from build123d import *

# Parameters (mm, degrees)
SKETCH_1_W          = 15.4
SKETCH_1_H          = 22.4
EXTRUDE_2_DEPTH     = 3
EXTRUDE_3_DEPTH     = 10
EXTRUDE_3_2_DEPTH   = 10
EXTRUDE_4_DEPTH     = 15
SKETCH_3_R          = 1.6
CUT_EXTRUDE_2_DEPTH = 31.8
SKETCH_9_R          = 1.3
SKETCH_9_R_2        = 3
SKETCH_9_R_3        = 1.55
CUT_EXTRUDE_6_DEPTH = 16
SKETCH_10_R         = 2.9
CUT_EXTRUDE_7_DEPTH = 2


with BuildPart() as part:
    # Sketch 1 → Extrude 2 (new body)
    with BuildSketch(Plane(origin=(0, 0, 0), x_dir=(1, 0, 0), z_dir=(0, 1, 0))):
        Rectangle(SKETCH_1_W, SKETCH_1_H)
    extrude(amount=EXTRUDE_2_DEPTH)



with BuildPart() as body_2:
    # Sketch 1_4 → Extrude 3 (new body)
    with BuildSketch(Plane(origin=(0, 0, 0), x_dir=(1, 0, 0), z_dir=(0, 1, 0))):
        Polygon((7.7, -11.2), (7.7, -7.7), (0, -7.7), (-4.7, -7.7), (-7.7, -7.7), (-7.7, -11.2), align=None)
    extrude(amount=EXTRUDE_3_DEPTH)


with BuildPart() as body_3:
    # Sketch 1_4 → Extrude 3 2 (new body)
    with BuildSketch(Plane(origin=(0, 0, 0), x_dir=(1, 0, 0), z_dir=(0, 1, 0))):
        Polygon((-7.7, 7.7), (0, 7.7), (7.7, 7.7), (7.7, 11.2), (-7.7, 11.2), align=None)
    extrude(amount=EXTRUDE_3_2_DEPTH)


with BuildPart() as part_1:
    add(part.part)

    add(body_2.part)  # Extrude 4 merges body 2

    add(body_3.part)  # Extrude 4 merges body 3
    # Sketch 1_5 → Extrude 4 (add)
    with BuildSketch(Plane(origin=(0, 0, 0), x_dir=(1, 0, 0), z_dir=(0, 1, 0))):
        Polygon((-7.7, 0), (-7.7, 7.7), (-7.7, 11.2), (-13.2, 11.2), (-13.2, -11.2), (-7.7, -11.2), (-7.7, -7.7), align=None)
        Polygon((7.7, 11.2), (7.7, 7.7), (7.7, 0), (7.7, -7.7), (7.7, -11.2), (13.2, -11.2), (13.2, 11.2), align=None)
        Polygon((7.7, -11.2), (7.7, -7.7), (0, -7.7), (-4.7, -7.7), (-7.7, -7.7), (-7.7, -11.2), align=None)
        Polygon((-7.7, 7.7), (0, 7.7), (7.7, 7.7), (7.7, 11.2), (-7.7, 11.2), align=None)
    extrude(amount=EXTRUDE_4_DEPTH)

    # Sketch 3 → Cut-Extrude 2 (cut, through all)
    with BuildSketch(Plane(origin=(0, 0, -19.6), x_dir=(-1, 0, 0), z_dir=(0, 0, -1))):
        with Locations((0, 3)):
            Circle(SKETCH_3_R)
        with Locations((-10, 3)):
            Circle(SKETCH_3_R)
        with Locations((10, 3)):
            Circle(SKETCH_3_R)
    extrude(amount=-CUT_EXTRUDE_2_DEPTH, mode=Mode.SUBTRACT)

    # Sketch 9 → Cut-Extrude 6 (cut, through all)
    with BuildSketch(Plane.XZ):
        with Locations((-4.949747468, -4.949747468)):
            Circle(SKETCH_9_R)
        with Locations((4.949747468, -4.949747468)):
            Circle(SKETCH_9_R)
        with Locations((4.949747468, 4.949747468)):
            Circle(SKETCH_9_R)
        with Locations((-4.949747468, 4.949747468)):
            Circle(SKETCH_9_R)
        Circle(SKETCH_9_R_2)
        with Locations((7, 0)):
            Circle(SKETCH_9_R_3)
        with Locations((0, 7)):
            Circle(SKETCH_9_R_3)
        with Locations((0, -7)):
            Circle(SKETCH_9_R_3)
        with Locations((-7, 0)):
            Circle(SKETCH_9_R_3)
    extrude(amount=-CUT_EXTRUDE_6_DEPTH, mode=Mode.SUBTRACT)

    # Sketch 10 → Cut-Extrude 7 (cut)
    with BuildSketch(Plane(origin=(0, 0, -11.2), x_dir=(-1, 0, 0), z_dir=(0, 0, -1))):
        with Locations((10, 3)):
            Circle(SKETCH_10_R)
        with Locations((0, 3)):
            Circle(SKETCH_10_R)
        with Locations((-10, 3)):
            Circle(SKETCH_10_R)
    extrude(amount=-CUT_EXTRUDE_7_DEPTH, mode=Mode.SUBTRACT)


solid = part_1.part
Can you work these out from the model? Positions are in its coordinate system, mm. A direction names the side the tool comes from. Give positions to 0.01 mm unless a question says otherwise; leave off trailing zeros. Loops run counter-clockwise (first coordinate to the right, second up) from the corner with the lowest first, then second, coordinate; pieces in that order, holes last. Notation, with made-up numbers: (72, 65) -> (101, 65) arc R13 ccw to (101, 88) -> close; hole circle Ø7 at (-38.75, 5). An arc over 180 degrees is marked (long way). Return JSON: item names as keys, results as strings.
Q1. For pin 1 Ø1.5 at (x, y) = (9.5, 4.5) entering from -Z; pin 2 Ø1.9 at (x, y) = (0, 3) entering from -Z; pin 3 Ø3 at (x, z) = (5.5, -1.5) entering from +Y, each with a flat end and sliding along its axis, tell me the tip position at first contact or that it passes through.
Checks:
{"pin 1": "stops at z = -9.2", "pin 2": "passes through", "pin 3": "stops at y = 3"}
Q2. I need wall thicknesses on probe 1 along Z at (x, y) = (6, 5); probe 2 along X at (y, z) = (12.5, -4.75); probe 3 along X at (y, z) = (14, 0). Which ranges of each line are inside material? Lowest first, please.
Checks:
{"probe 1": "z = -11.2 to -7.7, 7.7 to 11.2", "probe 2": "x = -13.2 to -7.7, 7.7 to 13.2", "probe 3": "x = -13.2 to -8.55, 8.55 to 13.2"}
Q3. We'd pull the mould along Z, two halves only. Please class faces 1 (the face through (13.2, 7, 0)), 2 (the face through (-11.25, 1.75, -9.2)), 3 (the face through (-1.14, 0.99, -5.95)): released by +Z, released by -Z, zero draft, split by the parting line, or undercut.
Checks:
{"face 1": "zero draft", "face 2": "released by -Z", "face 3": "undercut"}
Q4. On a 3-axis mill with a long thin cutter (end or side, diameter ignored), from which of +Z, -Z, +X, -X, +Y, -Y can I reach the whole of each face in a straight line? I mean faces 4 (the face through (-5, 3, 0)), 5 (the face through (-0.02, 9.32, -8.55)), 6 (the face through (0.378, 5.875, -10.214)). Say none if no direction works.
Checks:
{"face 4": "+Y", "face 5": "+Y, -Y", "face 6": "-Z"}
Q5. I want a section at D-D, the plane z = 9. List the corners of the cut face in (x, y) for me.
Checks:
{"outline": "(-13.2, 0) -> (13.2, 0) -> (13.2, 15) -> (-13.2, 15) -> close; hole circle Ø3.2 at (-10, 3); hole circle Ø3.2 at (0, 3); hole circle Ø3.2 at (10, 3)"}
Q6. I want a section at B-B, the plane x = 0. List the corners of the cut face in (y, z) for me.
Checks:
{"outline": "(0, -11.2) -> (0.1, -11.2) -> (0.1, -9.2) -> (1.4, -9.2) -> (1.4, -8.55) -> (0, -8.55) -> close; (0, -5.45) -> (1.4, -5.45) -> (1.4, -3) -> (0, -3) -> close; (0, 3) -> (1.4, 3) -> (1.4, 5.45) -> (0, 5.45) -> close; (0, 8.55) -> (1.4, 8.55) -> (1.4, 11.2) -> (0, 11.2) -> close; (4.6, -9.2) -> (5.9, -9.2) -> (5.9, -11.2) -> (15, -11.2) -> (15, -8.55) -> (4.6, -8.55) -> close; (4.6, 8.55) -> (15, 8.55) -> (15, 11.2) -> (4.6, 11.2) -> close"}
Q7. I want a section at C-C, the plane y = 13. List the corners of the cut face in (x, z) for me, then the cut area to 3 significant figures.
Checks:
{"outline": "(-13.2, -11.2) -> (13.2, -11.2) -> (13.2, 11.2) -> (-13.2, 11.2) -> close; hole (-7.7, -7.7) -> (-1.38, -7.7) arc R1.55 ccw to (1.38, -7.7) -> (7.7, -7.7) -> (7.7, -1.38) arc R1.55 ccw to (7.7, 1.38) -> (7.7, 7.7) -> (1.38, 7.7) arc R1.55 ccw to (-1.38, 7.7) -> (-7.7, 7.7) -> (-7.7, 1.38) arc R1.55 ccw to (-7.7, -1.38) -> close", "area": "347 mm2"}
Q8. I want a section at A-A, the plane z = -7. List the corners of the cut face in (x, y) for me, then the cut area to 3 significant figures.
Checks:
{"outline": "(-13.2, 0) -> (-1.55, 0) -> (-1.55, 2.6) arc R1.6 cw to (-1.6, 3) -> (-7.7, 3) -> (-7.7, 15) -> (-13.2, 15) -> close; (1.55, 0) -> (13.2, 0) -> (13.2, 15) -> (7.7, 15) -> (7.7, 3) -> (1.6, 3) arc R1.6 cw to (1.55, 2.6) -> close; hole circle Ø3.2 at (-10, 3); hole circle Ø3.2 at (10, 3)", "area": "186 mm2"}
